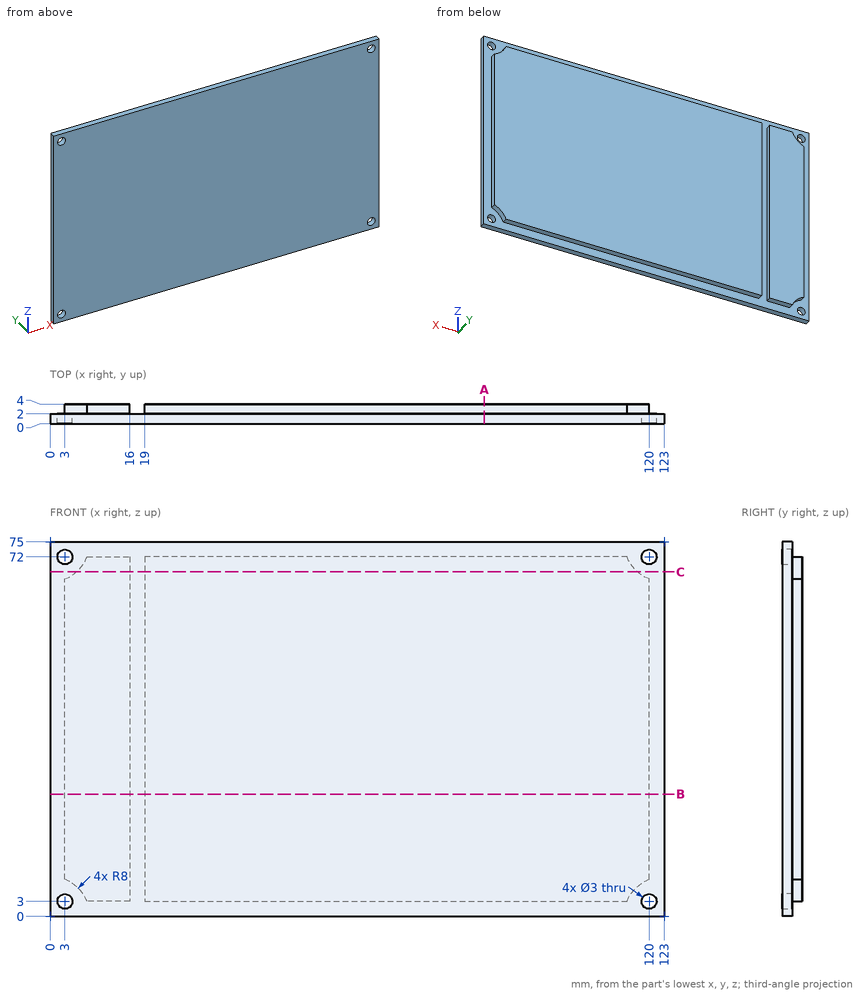
For this review, use the dimensioned drawing (mm, ordinates from the lowest corner) and the shaded views. Coordinates: 2 decimals unless noted, no trailing zeros. Write each loop counter-clockwise with the first axis right and the second up, starting at its lowest first coordinate (ties: lowest second). Pieces come first, ordered by that corner, then holes. Notation, with made-up numbers: (-4.75, 52) - (2.25, 52) arc R23 cw to (2.25, 87) - close; hole circle Ø7 at (-6.5, 55.5). An arc over 180 degrees is marked (long way). One line per item, written item: value.
1) To check wall thickness, follow probe 1 along X at (y, z) = (0.6, 3); probe 2 along Z at (x, y) = (120, 0.9); probe 3 along X at (y, z) = (0.4, 71.5). State the ranges of each line that lie inside material, in increasing order.
Answer sheet:
probe 1: x = 0 to 1.5, 4.5 to 118.5, 121.5 to 123
probe 2: z = 0 to 1.5, 4.5 to 70.5, 73.5 to 75
probe 3: x = 0 to 1.59, 4.41 to 118.59, 121.41 to 123
2) Add section A-A (x = 87). State the section outline as (y, z) points.
Answer sheet:
outline: (0, 0) - (2, 0) - (2, 3) - (4, 3) - (4, 72) - (2, 72) - (2, 75) - (0, 75) - close
3) Add section B-B (z = 24.5). State the section outline as (x, y) points.
Answer sheet:
outline: (0, 0) - (123, 0) - (123, 2) - (120, 2) - (120, 4) - (19, 4) - (19, 2) - (16, 2) - (16, 4) - (3, 4) - (3, 2) - (0, 2) - close
4) Insertion check: pin 1 (2.5 mm diameter, centred on x = 120, z = 72, fed in from -Y); pin 2 (0.6 mm diameter, centred on y = 3, z = 47.5, fed in from -X); pin 3 (1.6 mm diameter, centred on x = 53.5, y = 3.5, fed in from +Z); pin 4 (0.6 mm diameter, centred on y = 3, z = 37.5, fed in from +X). Each pin has a flat end and moves straight along its axis. Give the tip position at first contact, or say it passes through.
Answer sheet:
pin 1: passes through
pin 2: stops at x = 3
pin 3: stops at z = 72
pin 4: stops at x = 120
5) Add section C-C (z = 69). State the section outline as (x, y) points.
Answer sheet:
outline: (0, 0) - (123, 0) - (123, 2) - (117.71, 2) - (117.71, 4) - (19, 4) - (19, 2) - (16, 2) - (16, 4) - (5.29, 4) - (5.29, 2) - (0, 2) - close
